Geometry check sheet. Reference: the model listing, model coordinates, mm. Face numbers are marked on the shaded views. Round coordinates to 2 decimals unless told otherwise and drop trailing zeros. Write each loop counter-clockwise with the first axis right and the second up, starting at its lowest first coordinate (ties: lowest second). Pieces come first, ordered by that corner, then holes. Notation, with made-up numbers: M 55,72 L 96,72 A25 ccw 96,106 Z; hole C -37,-27 d7. An arc over 180 degrees is marked long. One line per item, written item: value. Start each with the question number.
1. Section check B-B (y = -39). Record the boundary of the cut face in (x, z).
2. Release check for a two-part mould opening along X. For the marked faces 1, 2, 3 and 4 record: pulls with the +X half, pulls with the -X half, needs draft (parallel to the pull), parting line crosses it, or undercut.
3. Section check A-A (z = 150.5). Record the boundary of the cut face in (x, y), and give its area (3 significant figures).
4. Section check C-C (x = -59). Record the boundary of the cut face in (y, z), and give its area (3 significant figures).
5. Scan lines: probe 1 along Z at (x, y) = (-36, 2); probe 2 along X at (y, z) = (-4, 109); probe 3 along Y at (x, z) = (-90.5, 308.5). Record each from-to range of solid material in increasing order. Write a range as [from, to].
6. Depth check by flat-ended pin: P1, Ø4, axis at x = -126, z = 39, coming from the -Y side. Enter the tip coordinate at first touch or a pass-through.
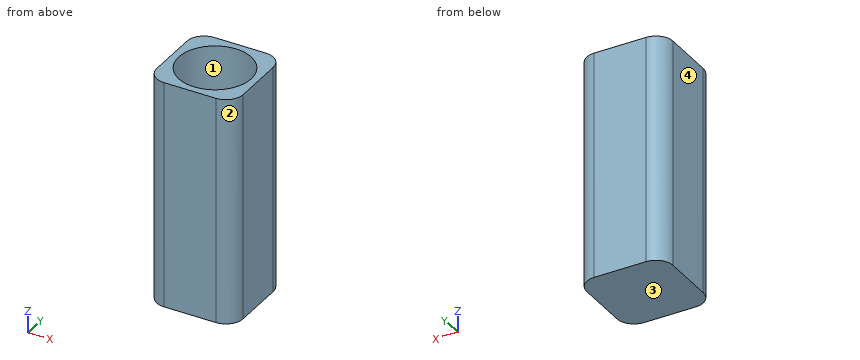
from build123d import *

# Parameters (mm, degrees)
F0_W     = 127
F0_H     = 127
F1_DEPTH = 335.28
F2_R     = 53.34
F3_DEPTH = 309.88
F4_R     = 25.4


with BuildPart() as f1:
    # F0 (on Top) → F1 (new body)
    with BuildSketch(Plane.XY):
        with Locations((-83.174668, -4.380767)):
            Rectangle(F0_W, F0_H)
    extrude(amount=F1_DEPTH)

    # F2 (on face) → F3 (cut)
    with BuildSketch(Plane.XY.offset(335.28)):
        with Locations((-83.174668, -4.380767)):
            Circle(F2_R)
    extrude(amount=-F3_DEPTH, mode=Mode.SUBTRACT)

    # F4
    f4_edges = [f1.edges().sort_by_distance(p)[0] for p in [
        (-19.674668, 59.119233, 167.64),
        (-146.674668, 59.119233, 167.64),
        (-146.674668, -67.880767, 167.64),
        (-19.674668, -67.880767, 167.64),
    ]]
    fillet(f4_edges, radius=F4_R)


solid = f1.part
Result sheet:
1. outline: M -146.67,0 L -19.67,0 L -19.67,335.28 L -42.6,335.28 L -42.6,25.4 L -123.75,25.4 L -123.75,335.28 L -146.67,335.28 Z
2. face 1: undercut
2. face 2: pulls with the +X half
2. face 3: needs draft
2. face 4: pulls with the -X half
3. outline: M -146.67,-42.48 A25.4 ccw -121.27,-67.88 L -45.07,-67.88 A25.4 ccw -19.67,-42.48 L -19.67,33.72 A25.4 ccw -45.07,59.12 L -121.27,59.12 A25.4 ccw -146.67,33.72 Z; hole C -83.17,-4.38 d106.68
3. area: 6,640 mm2
4. outline: M -67.88,0 L 59.12,0 L 59.12,335.28 L 43.17,335.28 L 43.17,25.4 L -51.93,25.4 L -51.93,335.28 L -67.88,335.28 Z
4. area: 13,100 mm2
5. probe 1: z = [0, 25.4]
5. probe 2: x = [-146.67, -136.51], [-29.84, -19.67]
5. probe 3: y = [-67.88, -57.22], [48.45, 59.12]
6. P1: stops at y = -67.73
